The listing builds one solid part. Answer for the finished solid, in the listing's coordinates (mm). Face numbers are marked on the shaded views. A direction names the side the tool comes from. Coordinates: 2 decimals unless noted, no trailing zeros. Loops run counter-clockwise (first coordinate to the right, second up) from the corner with the lowest first, then second, coordinate; pieces in that order, holes last. Notation, with made-up numbers: (-25, 83.5) -> (-7, 83.5) arc R32 cw to (-7, 119.5) -> close; hole circle Ø5 at (43.25, 0.5). An arc over 180 degrees is marked (long way). Answer in a Markdown table with one row per item.
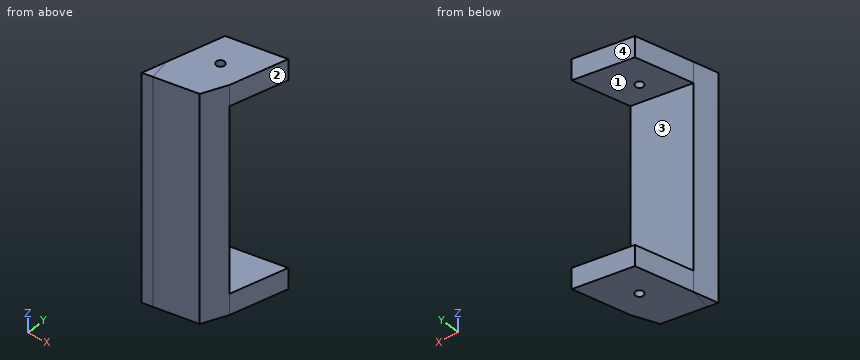
Autodesk Inventor part; units mm, degrees
ref_plane "YZ Plane" through (0, 0, 0) normal (1, 0, 0) x (0, 1, 0)
ref_plane "XZ Plane" through (0, 0, 0) normal (0, 1, 0) x (-1, 0, 0)
ref_plane "XY Plane" through (0, 0, 0) normal (0, 0, 1) x (1, 0, 0)
ref_plane "작업 평면1" through (0, 0, 0) normal (0, 0, 1) x (1, 0, 0)
sketch "스케치1" plane through (0, 0, 0) normal (0, 0, 1) x (1, 0, 0)
  circle A0 centre (5.0902, -34.5274) radius 1.15
  arc A1 (-17.0321, 89.7044) -> (-16.6881, 73.0594) centre (-9.9807, 81.5241) ccw
  line L0 (-16.6881, 73.0594) -> (-0.201, -26.5164)
  line L1 (-0.201, -26.5164) -> (-4.4157, -41.6132)
  line L2 (-4.4157, -41.6132) -> (11.3694, -38.9996)
  line L3 (11.3694, -38.9996) -> (15.5841, -23.9028)
  line L4 (15.5841, -23.9028) -> (-0.903, 75.673)
  arc A2 (-0.903, 75.673) -> (-5.9423, 91.5406) centre (-9.9807, 81.5241) ccw
  arc A3 (-5.9423, 91.5406) -> (-7.3028, 90.4498) centre (-6.3162, 90.6132) ccw
  line L5 (-7.3028, 90.4498) -> (-5.9358, 82.1938)
  arc A4 (-14.0257, 80.8544) -> (-5.9358, 82.1938) centre (-9.9807, 81.5241) ccw
  line L6 (-14.0257, 80.8544) -> (-15.3926, 89.1104)
  arc A5 (-15.3926, 89.1104) -> (-17.0321, 89.7044) centre (-16.3792, 88.947) ccw
  circle A6 centre (-14.6376, 75.0192) radius 1.3
  circle A7 centre (-3.4758, 76.8673) radius 1.3
  circle A8 centre (-5.3239, 88.029) radius 1.3
  circle A9 centre (-8.6739, 73.6316) radius 1.3
  circle A10 centre (-2.0882, 82.8309) radius 1.3
  circle A11 centre (-16.4857, 86.1809) radius 1.3
  circle A12 centre (-17.8733, 80.2173) radius 1.3
  line L7 (-0.201, -26.5164) -> (15.5841, -23.9028)
  point P0 (0, 0)
extrude "돌출1" add sketch "스케치1" along normal blind 6 contours L7 L3 L2 L1
ref_plane "작업 평면2" through (0, 0, -53) normal (0, 0, -1) x (-1, 0, 0)
sketch "스케치2" plane through (0, 0, -53) normal (0, 0, -1) x (-1, 0, 0)
  line L0 (4.4157, -41.6132) -> (-11.3694, -38.9996)
  line L1 (-11.3694, -38.9996) -> (-15.5841, -23.9028)
  line L2 (-15.5841, -23.9028) -> (0.201, -26.5164)
  line L3 (0.201, -26.5164) -> (4.4157, -41.6132)
  circle A0 centre (-5.0902, -34.5274) radius 1.15
  point P0 (0, 0)
extrude "돌출2" add sketch "스케치2" along normal blind 6
sketch "스케치7" plane through (-4.4157, -41.6132, -59) normal (0.1633496, -0.9865682, 0) x (0.9865682, 0.1633496, 0)
  line L0 (16, 6) -> (0, 6)
  line L1 (0, 6) -> (0, 0)
  line L2 (16, 0) -> (0, 0)
  line L3 (16, 6) -> (16, 0)
  line L4 (0, 59) -> (16, 59)
  line L5 (16, 59) -> (16, 65)
  line L6 (0, 65) -> (16, 65)
  line L7 (0, 59) -> (0, 65)
  line L8 (16, 0) -> (0, 0)
  line L9 (0, 0) -> (16, 0)
  line L10 (16, 0) -> (16, 65)
  line L11 (16, 65) -> (0, 65)
  line L12 (0, 65) -> (0, 0)
  point P0 (11.1539, 59)
  point P1 (16, 6)
  point P2 (16, 59)
  point P3 (0, 6)
extrude "돌출4" add sketch "스케치7" along normal blind 6
sketch "스케치8" plane through (0, 0, 6) normal (0, 0, 1) x (1, 0, 0)
  line L0 (11.3694, -38.9996) -> (15.5841, -23.9028)
  line L1 (15.5841, -23.9028) -> (-0.201, -26.5164)
  line L2 (-0.201, -26.5164) -> (-4.4157, -41.6132)
  line L3 (-4.4157, -41.6132) -> (-3.4356, -47.5326)
  line L4 (12.3495, -44.919) -> (-3.4356, -47.5326)
  line L5 (11.3694, -38.9996) -> (12.3495, -44.919)
  circle A0 centre (5.0902, -34.5274) radius 1.15
  line L6 (11.3694, -38.9996) -> (8.2961, -45.5901)
  line L7 (11.3694, -38.9996) -> (19.8926, -38.9996) construction
  point P0 (0, 0)
  dimension "d8" = 115
extrude "돌출5" cut sketch "스케치8" against normal blind 70 contours L5 L4 L6
sketch "스케치9" plane through (0, 0, 6) normal (0, 0, 1) x (1, 0, 0)
  circle A0 centre (5.0902, -34.5274) radius 1.15
  line L0 (8.2961, -45.5901) -> (11.3694, -38.9996)
  line L1 (11.3694, -38.9996) -> (15.5841, -23.9028)
  line L2 (15.5841, -23.9028) -> (-0.201, -26.5164)
  line L3 (-0.201, -26.5164) -> (-4.4157, -41.6132)
  line L4 (-4.4157, -41.6132) -> (-3.4356, -47.5326)
  line L5 (8.2961, -45.5901) -> (-3.4356, -47.5326)
  line L6 (-4.4157, -41.6132) -> (-7.6705, -53.2716)
  line L7 (3.9402, -46.3113) -> (-21.3119, -50.4924)
  point P0 (0, 0)
  point P1 (-6.1959, -47.9896)
extrude "돌출6" add sketch "스케치9" against normal blind 65 contours L7 L6 L4
properties part number "70" material "LCP 플라스틱"
Item 1: A tool of negligible diameter and unlimited length cuts with its end or side. For the marked faces 3 and 4, from which of +Z, -Z, +X, -X, +Y, -Y can it reach the whole face along a straight path? Write none if from no direction.
Findings below:
| item | result |
|---|---|
| face 3 | -X, +Y |
| face 4 | +Z, -Z, -X, +Y |
Item 2: A cutting plane is placed at C-C, the plane z = -46.5. Determine the outline of the cut face in (x, y).
Findings below:
| item | result |
|---|---|
| outline | (-6.2, -47.99) -> (-3.44, -47.53) -> (8.3, -45.59) -> (11.37, -39) -> (-4.42, -41.61) -> close |
Item 3: Determine the mould class of the marked faces 1 and 2 for opening direction Z: +Z half, -Z half, draft (parallel to the pull), parting line (faces both ways), or undercut.
Findings below:
| item | result |
|---|---|
| face 1 | undercut |
| face 2 | draft |
Item 4: A cutting plane is placed at A-A, the plane y = -32.25. Determine the outline of the cut face in (x, z), plus the area to 3 significant figures.
Findings below:
| item | result |
|---|---|
| outline | (-1.8, -59) -> (13.25, -59) -> (13.25, -53) -> (-1.8, -53) -> close; (-1.8, 0) -> (13.25, 0) -> (13.25, 6) -> (-1.8, 6) -> close |
| area | 181 mm2 |
Item 5: Find the intervals of material crossed by probe 1 along Z at (x, y) = (2.75, -39.5); probe 2 along Y at (x, z) = (5, -54); probe 3 along Y at (x, z) = (7.5, -17), in increasing order.
Findings below:
| item | result |
|---|---|
| probe 1 | z = -59 to -53, 0 to 6 |
| probe 2 | y = -46.14 to -35.67, -33.38 to -25.66 |
| probe 3 | y = -45.72 to -39.64 |
Item 6: A cutting plane is placed at B-B, the plane x = 2. Determine the outline of the cut face in (y, z).
Findings below:
| item | result |
|---|---|
| outline | (-46.63, -59) -> (-26.15, -59) -> (-26.15, -53) -> (-40.55, -53) -> (-40.55, 0) -> (-26.15, 0) -> (-26.15, 6) -> (-46.63, 6) -> close |
Item 7: A flat-ended cylindrical pin translates along its axis: pin 1 Ø4 at (y, z) = (-26.5, -52) entering from -X. Find the tip coordinate at first contact, or state that the pin passes through.
Findings below:
| item | result |
|---|---|
| pin 1 | stops at x = -0.68 |
Item 8: A cutting plane is placed at D-D, the plane y = -41. Determine the outline of the cut face in (x, z).
Findings below:
| item | result |
|---|---|
| outline | (-4.24, -59) -> (10.44, -59) -> (10.44, 6) -> (-4.24, 6) -> (-4.24, 0) -> (-0.71, 0) -> (-0.71, -53) -> (-4.24, -53) -> close |
